Can you work these out from the model? Positions are in its coordinate system, mm. Coordinates: 2 decimals unless noted, no trailing zeros. Order: outer loops, then holes, each group sorted by start corner. A loop starts at its lowest first (then second) coordinate and runs counter-clockwise, first axis right, second up. Notation, with made-up numbers: (-27.75, -14) -> (23.25, -14) arc R30 cw to (23.25, 18) -> close; hole circle Ø6 at (23, 37.5). An arc over 180 degrees is marked (long way). Answer in a Markdown table with one row per item. Add a question column.
1. Imagine slicing it at D-D on y = 11. Write out the boundary of the cut face in (x, z).
2. Imagine slicing it at C-C on z = 1.8. Write out the boundary of the cut face in (x, y), plus the area to 3 significant figures.
3. Imagine slicing it at A-A on y = 0. State how many separate pieces and enclosed holes the cut face has, plus the area to 4 significant figures.
4. Will these pins go through, and if not, where does the flat tip stop? pin 1 (3 mm diameter, centred on x = 108.5, y = 0, fed in from -Z); pin 2 (1.5 mm diameter, centred on x = 29.5, z = 2.5, fed in from +Y); pin 3 (1.8 mm diameter, centred on x = 80.7, y = 0, fed in from +Z); pin 4 (1.5 mm diameter, centred on x = 54, z = 1.5, fed in from -Y).
5. If I drill on line 1 along Y through (x, z) = (50, 2.1); line 2 along Y through (x, z) = (0, 1.65); line 3 along X through (y, z) = (6, 0.2), over which ranges is the centre line in solid material (lowest first)? Write a range as [from, to].
6. Imagine slicing it at B-B on x = 80.7. Write out the boundary of the cut face in (y, z), plus the area to 3 significant figures.
from build123d import *

# Parameters (mm, degrees)
ESKIZ_KONTUR_W        = 23.2
ESKIZ_KONTUR_H        = 12.6
PLASTINA_DEPTH        = 3
OTVERSTIYA_DEPTH      = 116.156318141
OTVERSTIYA_DEPTH_BACK = 116.156318141
ESKIZ_OTVERSTIYA_R    = 1.65
ESKIZ_OTVERSTIYA_R_2  = 1.1


with BuildPart() as part:
    # Eskiz_kontur → Plastina (new body)
    with BuildSketch(Plane.XY):
        with BuildLine():
            Line((7.29115, -15.8573), (0.27924, -15.99756))
            ThreePointArc((0.27924, -15.99756), (-15.999996904, 0), (0.27924, 15.99756))
            Line((0.27924, 15.99756), (7.29115, 15.8573))
            ThreePointArc((7.29115, 15.8573), (46.200008227, 9.528004702), (85.330859965, 14.296198255))
            Line((85.330859965, 14.296198255), (100.244329965, 13.997868255))
            ThreePointArc((100.244329965, 13.997868255), (113.999902223, 0), (100.244329965, -13.997868255))
            Line((100.244329965, -13.997868255), (85.330859965, -14.296198255))
            ThreePointArc((85.330859965, -14.296198255), (46.200008227, -9.528004702), (7.29115, -15.8573))
        make_face()
        with BuildLine():
            Line((58, 3), (44, 3))
            ThreePointArc((44, 3), (41, 0), (44, -3))
            Line((44, -3), (58, -3))
            ThreePointArc((58, -3), (61, 0), (58, 3))
        make_face(mode=Mode.SUBTRACT)
        with Locations((94.6, 0)):
            Rectangle(ESKIZ_KONTUR_W, ESKIZ_KONTUR_H, mode=Mode.SUBTRACT)
    extrude(amount=PLASTINA_DEPTH)

    # Eskiz_otverstiya → Otverstiya (cut, two sides: drawn at the far end of the back side and taken through both)
    with BuildSketch(Plane.XY.offset(-OTVERSTIYA_DEPTH_BACK)):
        Circle(ESKIZ_OTVERSTIYA_R)
        with Locations((35, 0)):
            Circle(ESKIZ_OTVERSTIYA_R)
        with Locations((68, 0)):
            Circle(ESKIZ_OTVERSTIYA_R)
        with Locations((80.7, 0)):
            Circle(ESKIZ_OTVERSTIYA_R_2)
        with Locations((108.5, 0)):
            Circle(ESKIZ_OTVERSTIYA_R_2)
    extrude(amount=OTVERSTIYA_DEPTH + OTVERSTIYA_DEPTH_BACK, mode=Mode.SUBTRACT)


solid = part.part
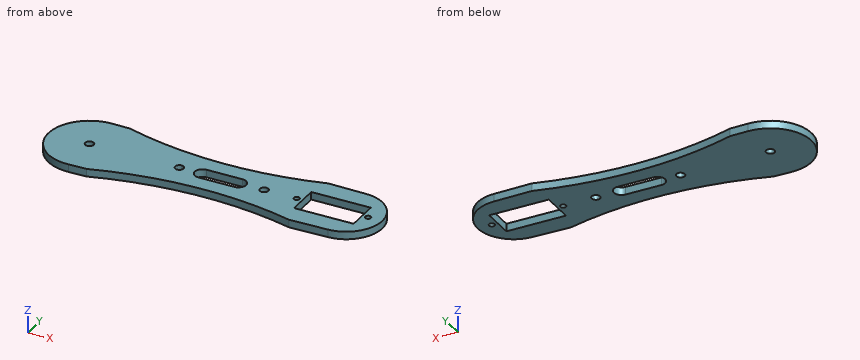
Answers follow:
| question | item | result |
|---|---|---|
| 1 | outline | (-11.62, 0) -> (28.56, 0) -> (28.56, 3) -> (-11.62, 3) -> close; (69.44, 0) -> (108.66, 0) -> (108.66, 3) -> (69.44, 3) -> close |
| 2 | outline | (0.28, -16) -> (7.29, -15.86) arc R140 cw to (85.33, -14.3) -> (100.24, -14) arc R14 ccw to (100.24, 14) -> (85.33, 14.3) arc R140 cw to (7.29, 15.86) -> (0.28, 16) arc R16 ccw (long way) to start; hole circle Ø3.3 at (0, 0); hole circle Ø3.3 at (35, 0); hole (44, -3) -> (58, -3) arc R3 ccw to (58, 3) -> (44, 3) arc R3 ccw to start; hole circle Ø3.3 at (68, 0); hole circle Ø2.2 at (80.7, 0); hole (83, -6.3) -> (106.2, -6.3) -> (106.2, 6.3) -> (83, 6.3) -> close; hole circle Ø2.2 at (108.5, 0) |
| 2 | area | 2,690 mm² |
| 3 | separate pieces | 8 |
| 3 | enclosed holes | 0 |
| 3 | area | 217.5 mm² |
| 4 | pin 1 | stops at z = 0 |
| 4 | pin 2 | stops at y = 10.97 |
| 4 | pin 3 | passes through |
| 4 | pin 4 | stops at y = -9.62 |
| 5 | line 1 | y = [-9.5, -3], [3, 9.5] |
| 5 | line 2 | y = [-16, -1.65], [1.65, 16] |
| 5 | line 3 | x = [-14.83, 83], [106.2, 112.65] |
| 6 | outline | (-13.14, 0) -> (-1.1, 0) -> (-1.1, 3) -> (-13.14, 3) -> close; (1.1, 0) -> (13.14, 0) -> (13.14, 3) -> (1.1, 3) -> close |
| 6 | area | 72.2 mm² |
